from build123d import *

# Parameters (mm, degrees)
SKETCH1_W           = 240
SKETCH1_H           = 200
BOSS_EXTRUDE1_DEPTH = 7.5
SKETCH4_R           = 2.6
CUT_EXTRUDE3_DEPTH  = 16
LPATTERN1_COUNT     = 8
LPATTERN1_PITCH     = 25
SKETCH5_R           = 1.5
CUT_EXTRUDE4_DEPTH  = 16


with BuildPart() as part:
    # Sketch1 → Boss-Extrude1 (new body, symmetric)
    with BuildSketch(Plane.XY):
        Rectangle(SKETCH1_W, SKETCH1_H)
    extrude(amount=BOSS_EXTRUDE1_DEPTH, both=True)

    # Sketch4 → Cut-Extrude3 (cut, through all)
    with BuildSketch(Plane.XY.offset(7.5)):
        with Locations((-110, 87.5)):
            Circle(SKETCH4_R)
        with Locations((110, 87.5)):
            Circle(SKETCH4_R)
    cut_extrude3 = extrude(amount=-CUT_EXTRUDE3_DEPTH, mode=Mode.SUBTRACT)

    # LPattern1: Cut-Extrude3 ×8
    with Locations(*[(0, -i * LPATTERN1_PITCH, 0) for i in range(1, LPATTERN1_COUNT)]):
        add(cut_extrude3, mode=Mode.SUBTRACT)

    # Sketch5 → Cut-Extrude4 (cut, through all)
    with BuildSketch(Plane.XY.offset(7.5)):
        with Locations((-95, 96.5)):
            Circle(SKETCH5_R)
        with Locations((-75, 96.5)):
            Circle(SKETCH5_R)
    extrude(amount=-CUT_EXTRUDE4_DEPTH, mode=Mode.SUBTRACT)


solid = part.part
Can you work these out from the model? Positions are in its coordinate system, mm. Coordinates: 2 decimals unless noted, no trailing zeros. Loops run counter-clockwise (first coordinate to the right, second up) from the corner with the lowest first, then second, coordinate; pieces in that order, holes last. Notation, with made-up numbers: (31.25, 2.25) - (51.25, 2.25) arc R16 ccw to (51.25, 30.25) - close; hole circle Ø9 at (88, -31.5). An arc over 180 degrees is marked (long way). Answer as a JSON object with one key per item and string values. Group by question number.
Item 1: If we section it at B-B (x = -110): State how many separate pieces and enclosed holes the cut face has, plus the area to 3 significant figures.
Item 2: If we section it at A-A (y = 62.5): List the corners of the cut face in (x, z) for me, plus the area to 3 significant figures.
Item 3: If I drill on L1, parallel to X at y = 96.5, z = -4; L2, parallel to X at y = -62, z = 4.25; L3, parallel to Y at x = -95, z = 1, over which ranges is the centre line in solid material (lowest first)? Write a range as from..to.
Item 4: If we mould it in two halves opening along X, with no side actions, what happens to faces 1 (the face through (120, -1, 0)), 2 (the face through (-2, 100, 0)), 3 (the face through (111.4, -85.31, 0.11))? For each: released by +X, released by -X, zero draft, split by the parting line, or undercut.
Returned:
{
 "1": {"separate pieces": "9", "enclosed holes": "0", "area": "2,380 mm²"},
 "2": {"outline": "(-120, -7.5) - (-112.6, -7.5) - (-112.6, 7.5) - (-120, 7.5) - close; (-107.4, -7.5) - (107.4, -7.5) - (107.4, 7.5) - (-107.4, 7.5) - close; (112.6, -7.5) - (120, -7.5) - (120, 7.5) - (112.6, 7.5) - close", "area": "3,440 mm²"},
 "3": {"L1": "x = -120..-96.5, -93.5..-76.5, -73.5..120", "L2": "x = -120..-112.55, -107.45..107.45, 112.55..120", "L3": "y = -100..95, 98..100"},
 "4": {"face 1": "released by +X", "face 2": "zero draft", "face 3": "undercut"}
}
